from build123d import *

# Parameters (mm, degrees)
SKETCH_W        = 64
SKETCH_H        = 100
PAD_DEPTH       = 22
PAD001_DEPTH    = 15
POCKET_DEPTH    = 100.001
SKETCH003_W     = 12
SKETCH003_H     = 70
PAD002_DEPTH    = 40
POCKET001_DEPTH = 12


with BuildPart() as part:
    # Sketch → Pad (new body)
    with BuildSketch(Plane.XY):
        Rectangle(SKETCH_W, SKETCH_H)
    extrude(amount=PAD_DEPTH)

    # Sketch001 (on Face1 of Pad) → Pad001 (join)
    with BuildSketch(Plane(origin=(0, 50, 0), x_dir=(-1, 0, 0), z_dir=(0, 1, 0))):
        Polygon((-32, 22), (-32, 59), (-16, 75), (16, 75), (32, 59), (32, 22), align=None)
    extrude(amount=-PAD001_DEPTH)

    # Sketch002 (on Face6 of Pad001) → Pocket (cut, through all)
    with BuildSketch(Plane.XZ.offset(50)):
        Polygon((-7.707092, 0), (-14.635295, 12), (15.364705, 12), (7.707092, 0), align=None)
    extrude(amount=-POCKET_DEPTH, mode=Mode.SUBTRACT)

    # Sketch003 (on Face12 of Pocket) → Pad002 (join)
    with BuildSketch(Plane.XY.offset(22)):
        Rectangle(SKETCH003_W, SKETCH003_H)
    extrude(amount=PAD002_DEPTH)

    # Sketch004 (on Face20 of Pad002) → Pocket001 (cut)
    with BuildSketch(Plane(origin=(-6, 0, 0), x_dir=(0, -1, 0), z_dir=(-1, 0, 0))):
        Polygon((-35, 62), (35, 22), (35, 62), align=None)
    extrude(amount=-POCKET001_DEPTH, mode=Mode.SUBTRACT)


solid = part.part
Build history of the part. All positions in model axes, mm. A direction names the side the tool comes from. Round coordinates to 2 decimals unless told otherwise and drop trailing zeros. Write each loop counter-clockwise with the first axis right and the second up, starting at its lowest first coordinate (ties: lowest second). Pieces come first, ordered by that corner, then holes. Notation, with made-up numbers: M 64,-23 L 89,-23 A22 cw 89,-8 Z; hole C 12.5,47.5 d8. An arc over 180 degrees is marked long. Answer as a JSON object with one key per item and string values. Group by question number.
(1) Drill centre lines: L1, parallel to X at y = 27.5, z = 10.5; L2, parallel to Z at x = 5, y = 36; L3, parallel to X at y = 2.5, z = 40.5. Where is each one in solid material? Low to high.
(2) Cut at A-A (x = 10.5). Give the cut face in (y, z), and give its area (3 significant figures).
(3) Mould opens along X. For faces 4 (the flat face through (-20, 1, 0)), 5 (the flat face through (0, -1, 12)), 6 (the flat face through (6, 15, 33)), 7 (the flat face through (-32, 12, 17)) say: pulls with the +X half, pulls with the -X half, needs draft (parallel to the pull), parting line crosses it, or undercut.
(4) Flat gauge pins, fed straight in: pin 1 (3 mm diameter, centred on x = -3, z = 46.5, fed in from -Y); pin 2 (19 mm diameter, centred on x = -1.5, y = -13.5, fed in from +Z); pin 3 (20 mm diameter, centred on y = 13, z = 47.5, fed in from -X). Where does each tip first touch, or does it go through?
(5) Cut at B-B (z = 8). Give the cut face in (x, y).
(6) Cut at D-D (y = -22). Give the cut face in (x, z).
(7) Cut at C-C (x = -19). Give the cut face in (y, z).
(8) Which spindle directions (+Z, -Z, +X, -X, +Y, -Y) get a long thin tool onto all of the face, cutting with end or side? Do faces 1 (the flat face through (-6, 15, 33)), 2 (the flat face through (-11.123, -0.7, 5.916)), 3 (the flat face through (-8, -7, 22)). Say none if no direction does.
Responses:
{
 "1": {"L1": "x = -32 to -13.77, 14.41 to 32", "L2": "z = 12 to 75", "L3": "x = -6 to 6"},
 "2": {"outline": "M -50,0 L 50,0 L 50,4.38 L -50,4.38 Z; M -50,12 L 50,12 L 50,75 L 35,75 L 35,22 L -50,22 Z", "area": "2,230 mm2"},
 "3": {"face 4": "needs draft", "face 5": "undercut", "face 6": "pulls with the +X half", "face 7": "pulls with the -X half"},
 "4": {"pin 1": "stops at y = 5.25", "pin 2": "stops at z = 39.71", "pin 3": "stops at x = -6"},
 "5": {"outline": "M -32,-50 L -12.33,-50 L -12.33,50 L -32,50 Z; M 12.81,-50 L 32,-50 L 32,50 L 12.81,50 Z"},
 "6": {"outline": "M -32,0 L -7.71,0 L -14.64,12 L 15.36,12 L 7.71,0 L 32,0 L 32,22 L 6,22 L 6,29.43 L -6,29.43 L -6,22 L -32,22 Z"},
 "7": {"outline": "M -50,0 L 50,0 L 50,72 L 35,72 L 35,22 L -50,22 Z"},
 "8": {"face 1": "+Z, -X, -Y", "face 2": "+Y, -Y", "face 3": "+Z, -Y"}
}
